Read the model definition and answer for the solid it produces. Units are mm, in the model's axes. A direction names the side the tool comes from. Coordinates: 2 decimals unless noted, no trailing zeros. Loops run counter-clockwise (first coordinate to the right, second up) from the corner with the lowest first, then second, coordinate; pieces in that order, holes last. Notation, with made-up numbers: (0, -12) -> (17, -12) arc R19 ccw to (17, 18) -> close; hole circle Ø7 at (63.25, -35). An arc over 180 degrees is marked (long way). Answer as a JSON object with one key per item and string values. Group by question number.
1) Section B-B, the plane x = -200 is taken. Give the vertices of the cut face in (y, z), plus the area to 3 significant figures.
2) Flat-ended cylindrical pins translate along their axes: P1, Ø0.6, axis at x = -40.5, y = 1.5, coming from the -Z side; P2, Ø6, axis at x = -66, z = 4, coming from the -Y side; P3, Ø1, axis at x = -185, y = 1.5, coming from the +Z side. Find the tip coordinate at first contact, or state that the pin passes through.
3) Section A-A, the plane z = 10 is taken. Give the vertices of the cut face in (x, y) (3 decimals), plus the area to 3 significant figures.
4) Which of the six approach directions +Z, -Z, +X, -X, +Y, -Y give full straight-line access (tool end or side, diameter ignored) to faces 5 (the face through (-19, 1, 18)), 6 (the face through (-110.31, 0.99, -19.91)), 7 (the face through (-18.5, 1.01, -60.97))?
5) Consider probe 1 along Z at (x, y) = (-10, 0.75) (3 decimals); probe 2 along Z at (x, y) = (-55.5, 0.4); probe 3 along X at (y, z) = (0.6, -38). Determine where each line is inside the solid, lowest interval first. Write a range as [from, to].
6) Determine the mould class of faces 1 (the face through (-1.43, 1.01, -60.9)), 2 (the face through (-223, 1, 18)), 3 (the face through (-206, 1, 19)), 4 (the face through (-211.877, 0.986, 9.907)) for opening direction X: released by +X, released by -X, zero draft, split by the parting line, or undercut.
Autodesk Inventor part; units mm, degrees
ref_plane "YZ Plane" through (0, 0, 0) normal (1, 0, 0) x (0, 1, 0)
ref_plane "XZ Plane" through (0, 0, 0) normal (0, 1, 0) x (-1, 0, 0)
ref_plane "XY Plane" through (0, 0, 0) normal (0, 0, 1) x (1, 0, 0)
sketch "Sketch1" plane through (0, 0, 0) normal (0, 1, 0) x (-1, 0, 0)
  line L0 (0, 0) -> (0, -42.4)
  line L1 (20, 0) -> (204, 0)
  line L2 (20, -42.4) -> (204, -42.4)
  line L3 (224, -42.4) -> (224, 0)
  line L4 (0, -42.4) -> (0, -62.4)
  line L5 (0, -62.4) -> (20, -62.4)
  line L6 (20, -62.4) -> (20, -42.4)
  line L7 (0, 0) -> (0, 20)
  line L8 (0, 20) -> (20, 20)
  line L9 (20, 20) -> (20, 0)
  line L10 (224, -42.4) -> (224, -62.4)
  line L11 (224, -62.4) -> (204, -62.4)
  line L12 (204, -62.4) -> (204, -42.4)
  line L13 (224, 0) -> (224, 20)
  line L14 (224, 20) -> (204, 20)
  line L15 (204, 20) -> (204, 0)
  circle A0 centre (10, -52.4) radius 2.125
  circle A1 centre (10, 10) radius 2.125
  circle A2 centre (214, -52.4) radius 2.125
  circle A3 centre (214, 10) radius 2.125
  circle A4 centre (112, -21.2) radius 2.125
  line L16 (0, -42.4) -> (0, -36.8)
  line L17 (0, -36.8) -> (8.4, -36.8)
  arc A5 (8.4, -35.2) -> (8.4, -38.4) centre (8.4, -36.8) ccw
  line L18 (0, 0) -> (0, -5.6)
  line L19 (0, -5.6) -> (8.4, -5.6)
  arc A6 (8.1881, -4.0141) -> (8.4, -7.2) centre (8.4, -5.6) ccw
  arc A7 (56.4, -38.4) -> (56.4, -35.2) centre (56.4, -36.8) ccw
  line L20 (8.4, -35.2) -> (56.4, -35.2)
  line L21 (56.4, -38.4) -> (8.4, -38.4)
  arc A8 (56.4, -7.2) -> (56.3995, -4) centre (56.4, -5.6) ccw
  line L22 (56.4, -7.2) -> (8.4, -7.2)
  line L23 (8.1881, -4.0141) -> (56.3995, -4)
  arc A9 (215.6, -38.4) -> (215.6, -35.2) centre (215.6, -36.8) ccw
  arc A10 (215.6, -7.2) -> (215.8119, -4.0141) centre (215.6, -5.6) ccw
  arc A11 (167.6, -35.2) -> (167.6, -38.4) centre (167.6, -36.8) ccw
  line L24 (215.6, -35.2) -> (167.6, -35.2)
  line L25 (167.6, -38.4) -> (215.6, -38.4)
  arc A12 (167.6005, -4) -> (167.6, -7.2) centre (167.6, -5.6) ccw
  line L26 (167.6, -7.2) -> (215.6, -7.2)
  line L27 (215.8119, -4.0141) -> (167.6005, -4)
  dimension "d1" = 42.4
  dimension "d2" = 224
  dimension "d3" = 224
  dimension "d4" = 20
  dimension "d5" = 20
  dimension "d6" = 20
  dimension "d7" = 20
  dimension "d8" = 20
  dimension "d9" = 20
  dimension "d10" = 4.25
  dimension "d11" = 4.25
  dimension "d12" = 4.25
  dimension "d13" = 4.25
  dimension "d14" = 4.25
  dimension "d15" = 5.6
  dimension "d16" = 8.4
  dimension "d17" = 3.2
  dimension "d18" = 5.6
  dimension "d19" = 3.2
  dimension "d23" = 3.2
  dimension "d28" = 3.2
extrude "Extrusion1" add sketch "Sketch1" along normal blind 2
fillet "Fillet1" radius 5 8 edges at (0, 1, 20) (-20, 1, 20) (0, 1, -62.4) (-20, 1, -62.4) (-204, 1, -62.4) (-224, 1, -62.4) (-204, 1, 20) (-224, 1, 20)
properties part number "Motor Attachment 3.0"
Determined:
{
 "1": {"outline": "(0, -42.4) -> (2, -42.4) -> (2, -38.4) -> (0, -38.4) -> close; (0, -35.2) -> (2, -35.2) -> (2, -7.2) -> (0, -7.2) -> close; (0, -4.01) -> (2, -4.01) -> (2, 0) -> (0, 0) -> close", "area": "72.0 mm²"},
 "2": {"P1": "z = -42.4", "P2": "through", "P3": "z = 0"},
 "3": {"outline": "(-224, 0) -> (-216.125, 0) -> (-216.125, 2) -> (-224, 2) -> close; (-211.875, 0) -> (-204, 0) -> (-204, 2) -> (-211.875, 2) -> close; (-20, 0) -> (-12.125, 0) -> (-12.125, 2) -> (-20, 2) -> close; (-7.875, 0) -> (0, 0) -> (0, 2) -> (-7.875, 2) -> close", "area": "63.0 mm²"},
 "4": {"face 5": "+Z, +Y, -Y", "face 6": "+Y, -Y", "face 7": "-Z, +Y, -Y"},
 "5": {"probe 1": "[-62.4, -54.525], [-50.275, -38.4], [-35.2, -7.2], [-4.014, 7.875], [12.125, 20]", "probe 2": "[-42.4, -38.4], [-35.2, -7.2], [-4, 0]", "probe 3": "[-224, -216.66], [-166.54, -57.46], [-7.34, 0]"},
 "6": {"face 1": "released by +X", "face 2": "released by -X", "face 3": "undercut", "face 4": "undercut"}
}
